from build123d import *

# Parameters (mm, degrees)
F0_R      = 15
F0_R_2    = 40
F1_DEPTH  = 10
F3_DEPTH  = 6.35
F5_DEPTH  = 6.35
F6_R      = 40
F6_R_2    = 15
F7_DEPTH  = 6.35
F8_R      = 40.1872824047
F8_R_2    = 15
F9_DEPTH  = 6.35
F10_R     = 3.175
F11_DEPTH = 24.638


with BuildPart() as f1:
    # F0 (on Front) → F1 (new body, symmetric)
    with BuildSketch(Plane.XZ):
        with BuildLine():
            Line((-38.1, 238.1), (-50.8, 238.1))
            Line((-50.8, 238.1), (-50.8, 161.9))
            Line((-50.8, 161.9), (-34.8479530832, 161.9))
            ThreePointArc((-34.8479530832, 161.9), (-21.3567895263, 146.9813784556), (-19.05, 127))
            Line((-19.05, 127), (-19.05, 0))
            ThreePointArc((-19.05, 0), (0, -19.05), (19.05, 0))
            Line((19.05, 0), (19.05, 127))
            ThreePointArc((19.05, 127), (21.3567895263, 146.9813784556), (34.8479530832, 161.9))
            Line((34.8479530832, 161.9), (50.8, 161.9))
            Line((50.8, 161.9), (50.8, 238.1))
            Line((50.8, 238.1), (38.1, 238.1))
            ThreePointArc((38.1, 238.1), (0, 253.8815367264), (-38.1, 238.1))
        make_face()
        Circle(F0_R, mode=Mode.SUBTRACT)
        with Locations((0, 200)):
            Circle(F0_R_2, mode=Mode.SUBTRACT)
    extrude(amount=F1_DEPTH, both=True)

    # F2 (on face) → F3 (cut)
    with BuildSketch(Plane(origin=(0, 10, 0), x_dir=(-1, 0, 0), z_dir=(0, 1, 0))):
        with BuildLine():
            Line((8.5645674547, 152.4), (-8.5645674547, 152.4))
            ThreePointArc((-8.5645674547, 152.4), (-13.165442891, 150.4265791688), (-14.9066448066, 145.7328961324))
            Line((-14.9066448066, 145.7328961324), (-9.1916448066, 31.4328961324))
            ThreePointArc((-9.1916448066, 31.4328961324), (-7.2261466235, 27.1491245638), (-2.8495674547, 25.4))
            Line((-2.8495674547, 25.4), (2.8495674547, 25.4))
            ThreePointArc((2.8495674547, 25.4), (7.2261466235, 27.1491245638), (9.1916448066, 31.4328961324))
            Line((9.1916448066, 31.4328961324), (14.9066448066, 145.7328961324))
            ThreePointArc((14.9066448066, 145.7328961324), (13.165442891, 150.4265791688), (8.5645674547, 152.4))
        make_face()
    extrude(amount=-F3_DEPTH, mode=Mode.SUBTRACT)

    # F4 (on face) → F5 (cut)
    with BuildSketch(Plane.XZ.offset(10)):
        with BuildLine():
            Line((8.5598, 152.4), (-8.5693349095, 152.4))
            ThreePointArc((-8.5693349095, 152.4), (-13.1702103457, 150.4265791688), (-14.9114122614, 145.7328961324))
            Line((-14.9114122614, 145.7328961324), (-9.1964122614, 31.4328961324))
            ThreePointArc((-9.1964122614, 31.4328961324), (-7.2309140782, 27.1491245638), (-2.8543349095, 25.4))
            Line((-2.8543349095, 25.4), (2.8448, 25.4))
            ThreePointArc((2.8448, 25.4), (7.2213791688, 27.1491245638), (9.1868773519, 31.4328961324))
            Line((9.1868773519, 31.4328961324), (14.9018773519, 145.7328961324))
            ThreePointArc((14.9018773519, 145.7328961324), (13.1606754362, 150.4265791688), (8.5598, 152.4))
        make_face()
    extrude(amount=-F5_DEPTH, mode=Mode.SUBTRACT)

    # F6 (on face) → F7 (join, symmetric)
    with BuildSketch(Plane.XZ.offset(10)):
        with BuildLine():
            ThreePointArc((8.1649718925, 152.4), (36.9239471908, 168.8704498932), (48.295204379, 200))
            ThreePointArc((48.295204379, 200), (-31.1295501068, 236.9239471908), (-8.1649718925, 152.4))
            Line((-8.1649718925, 152.4), (8.1649718925, 152.4))
        make_face()
        with Locations((0, 200)):
            Circle(F6_R, mode=Mode.SUBTRACT)
        with BuildLine():
            Line((19.05, 0), (19.05, 2.2343365964))
            ThreePointArc((19.05, 2.2343365964), (0, 19.1805828907), (-19.05, 2.2343365964))
            Line((-19.05, 2.2343365964), (-19.05, 0))
            ThreePointArc((-19.05, 0), (0, -19.05), (19.05, 0))
        make_face()
        Circle(F6_R_2, mode=Mode.SUBTRACT)
    extrude(amount=F7_DEPTH, both=True)

    # F8 (on face) → F9 (join, symmetric)
    with BuildSketch(Plane(origin=(0, 10, 0), x_dir=(-1, 0, 0), z_dir=(0, 1, 0))):
        with BuildLine():
            ThreePointArc((8.5645674547, 152.4), (37.1034478409, 168.976686605), (48.364365143, 200))
            ThreePointArc((48.364365143, 200), (-31.023313395, 237.1034478409), (-8.5645674547, 152.4))
            Line((-8.5645674547, 152.4), (8.5645674547, 152.4))
        make_face()
        with Locations((0, 200)):
            Circle(F8_R, mode=Mode.SUBTRACT)
        with BuildLine():
            Line((19.05, 0), (19.05, 1.2599718654))
            ThreePointArc((19.05, 1.2599718654), (0, 19.091621961), (-19.05, 1.2599718654))
            Line((-19.05, 1.2599718654), (-19.05, 0))
            ThreePointArc((-19.05, 0), (0, -19.05), (19.05, 0))
        make_face()
        Circle(F8_R_2, mode=Mode.SUBTRACT)
    extrude(amount=F9_DEPTH, both=True)

    # F10 (on face) → F11 (cut)
    with BuildSketch(Plane.XY.offset(238.1)):
        with Locations((-44.45, 0)):
            Circle(F10_R)
        with Locations((44.45, 0)):
            Circle(F10_R)
    extrude(amount=-F11_DEPTH, mode=Mode.SUBTRACT)


solid = f1.part
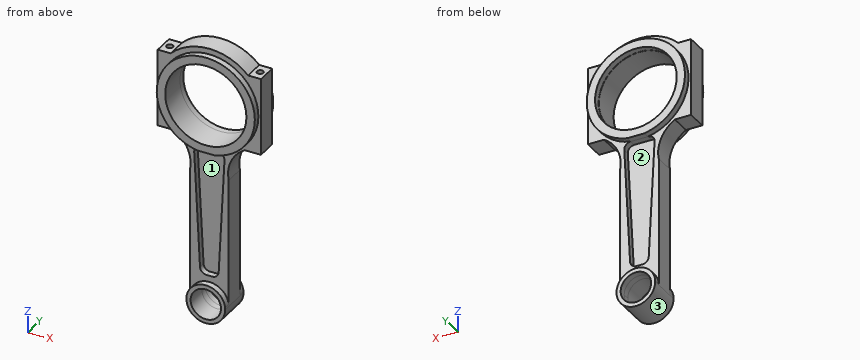
For this review, take the finished solid that the model builds, in its own axes (mm). Face numbers are marked on the shaded views. Give positions to 0.01 mm unless a question says otherwise; leave off trailing zeros. Loops run counter-clockwise (first coordinate to the right, second up) from the corner with the lowest first, then second, coordinate; pieces in that order, holes last. Notation, with made-up numbers: M 6.25,26 L 38.25,26 A22 cw 38.25,53 Z; hole C 43,-21 d3. An arc over 180 degrees is marked long. Put each result on its own line as item: value. Start each with the question number.
(1) Add section B-B, the plane x = 0. Give the number of separate pieces and of enclosed holes in the cut face, then the cut area to 3 significant figures.
(2) Add section D-D, the plane z = 205. Write out the cut boundary in (x, y), then the cut area to 3 significant figures.
(3) Wall thickness on L1, parallel to Z at x = 0, y = 15; L2, parallel to Z at x = 0, y = -11; L3, parallel to Z at x = 0, y = 2.75: over which ranges is each line inside the solid? List them lowest first.
(4) The part is to be moulded in two halves that separate along X. For the marked faces 1, 2 and 3, say which applies: +X half, -X half, draft (parallel to the pull), parting line (faces both ways), or undercut.
(5) For pin 1 (3 mm diameter, centred on y = -3.5, z = 143, fed in from +X); pin 2 (1 mm diameter, centred on y = 6, z = 151.5, fed in from +X); pin 3 (7 mm diameter, centred on x = 46, y = -1, fed in from +Z), all flat-tipped, find the tip position at first contact; note any pin that passes through.
(6) Add section A-A, the plane y = -7.5. Write out the cut boundary in (x, z).
(7) Add section C-C, the plane x = -25.5. Write out the cut boundary in (y, z), then the cut area to 3 significant figures.
Result:
1. separate pieces: 3
1. enclosed holes: 0
1. area: 1,950 mm^2
2. outline: M -50.8,-10 L -48.04,-10 L -48.04,-16.35 L -39.69,-16.35 L -39.69,10 L -39.88,10 L -39.88,16.35 L -48.11,16.35 L -48.11,10 L -50.8,10 Z; M 39.69,-16.35 L 48.04,-16.35 L 48.04,-10 L 50.8,-10 L 50.8,10 L 48.11,10 L 48.11,16.35 L 39.88,16.35 L 39.88,10 L 39.69,10 Z
2. area: 655 mm^2
3. L1: z = -19.05 to -15, 15 to 19.09, 152.4 to 159.81, 240.19 to 248.36
3. L2: z = -19.05 to -15, 15 to 19.18, 152.4 to 160, 240 to 248.3
3. L3: z = -19.05 to -15, 15 to 160, 240 to 253.88
4. face 1: undercut
4. face 2: undercut
4. face 3: parting line
5. pin 1: stops at x = 20.35
5. pin 2: stops at x = 24.18
5. pin 3: stops at z = 238.1
6. outline: M -50.8,161.9 L -34.85,161.9 A32.95 cw -19.05,127 L -19.05,0 A19.05 ccw 19.05,0 L 19.05,127 A32.95 cw 34.85,161.9 L 50.8,161.9 L 50.8,238.1 L 38.1,238.1 A53.88 ccw -38.1,238.1 L -50.8,238.1 Z; hole C 0,200 d80; hole C 0,0 d30; hole M -14.91,145.73 L -9.2,31.43 A6.35 ccw -2.85,25.4 L 2.84,25.4 A6.35 ccw 9.19,31.43 L 14.9,145.73 A6.35 ccw 8.56,152.4 L -8.57,152.4 A6.35 ccw Z
7. outline: M -16.35,158.99 L -10,158.99 L -10,153.79 L 10,153.79 L 10,158.9 L 16.35,158.9 L 16.35,168.94 L 10,168.94 L 10,169.18 L -16.35,169.18 Z; M -16.35,230.82 L 10,230.82 L 10,231.06 L 16.35,231.06 L 16.35,241.1 L 10,241.1 L 10,247.47 L -10,247.47 L -10,241.01 L -16.35,241.01 Z
7. area: 898 mm^2
